from build123d import *

# Parameters (mm, degrees)
SKETCH1_W           = 52
SKETCH1_H           = 25
BOSS_EXTRUDE1_DEPTH = 2
SKETCH3_R           = 4
SKETCH3_R_2         = 1.5
CUT_EXTRUDE1_DEPTH  = 3
SKETCH4_R           = 4
SKETCH4_R_2         = 1.5
BOSS_EXTRUDE3_DEPTH = 2
SKETCH5_R           = 4
SKETCH5_R_2         = 1.496339982
SKETCH5_R_3         = 1.5
BOSS_EXTRUDE4_DEPTH = 2


with BuildPart() as part:
    # Sketch1 → Boss-Extrude1 (new body)
    with BuildSketch(Plane(origin=(0, 0, 0), x_dir=(1, 0, 0), z_dir=(0, 1, 0))):
        Rectangle(SKETCH1_W, SKETCH1_H)
    extrude(amount=BOSS_EXTRUDE1_DEPTH)

    # Sketch3 → Cut-Extrude1 (cut, through all)
    with BuildSketch(Plane(origin=(0, 2, 0), x_dir=(1, 0, 0), z_dir=(0, 1, 0))):
        Circle(SKETCH3_R)
        with Locations((18.6, 0)):
            Circle(SKETCH3_R_2)
        with Locations((7, 0)):
            Circle(SKETCH3_R_2)
        with Locations((0, 7)):
            Circle(SKETCH3_R_2)
        with Locations((-7, 0)):
            Circle(SKETCH3_R_2)
        with Locations((0, -7)):
            Circle(SKETCH3_R_2)
        with Locations((-18.6, 0)):
            Circle(SKETCH3_R_2)
    extrude(amount=-CUT_EXTRUDE1_DEPTH, mode=Mode.SUBTRACT)

    # Sketch4 → Boss-Extrude3 (add)
    with BuildSketch(Plane(origin=(26, 0, 0), x_dir=(0, 0, -1), z_dir=(1, 0, 0))):
        with BuildLine():
            Line((-12.5, 0), (12.5, 0))
            Line((12.5, 0), (12.5, 32))
            ThreePointArc((12.5, 32), (0, 44.5), (-12.5, 32))
            Line((-12.5, 32), (-12.5, 0))
        make_face()
        with Locations((0, 32)):
            Circle(SKETCH4_R, mode=Mode.SUBTRACT)
        with Locations((0, 39)):
            Circle(SKETCH4_R_2, mode=Mode.SUBTRACT)
        with Locations((7, 32)):
            Circle(SKETCH4_R_2, mode=Mode.SUBTRACT)
        with Locations((0, 25)):
            Circle(SKETCH4_R_2, mode=Mode.SUBTRACT)
        with Locations((-7, 32)):
            Circle(SKETCH4_R_2, mode=Mode.SUBTRACT)
        with Locations((0, 13.4)):
            Circle(SKETCH4_R_2, mode=Mode.SUBTRACT)
    extrude(amount=BOSS_EXTRUDE3_DEPTH)

    # Sketch5 → Boss-Extrude4 (add)
    with BuildSketch(Plane.ZY.offset(26)):
        with BuildLine():
            Line((-12.5, 0), (12.5, 0))
            Line((12.5, 0), (12.5, 32))
            ThreePointArc((12.5, 32), (0, 44.5), (-12.5, 32))
            Line((-12.5, 32), (-12.5, 0))
        make_face()
        with Locations((0, 32)):
            Circle(SKETCH5_R, mode=Mode.SUBTRACT)
        with Locations((0, 39)):
            Circle(SKETCH5_R_2, mode=Mode.SUBTRACT)
        with Locations((7, 32)):
            Circle(SKETCH5_R_3, mode=Mode.SUBTRACT)
        with Locations((0, 25)):
            Circle(SKETCH5_R_3, mode=Mode.SUBTRACT)
        with Locations((-7, 32)):
            Circle(SKETCH5_R_3, mode=Mode.SUBTRACT)
        with Locations((0, 13.4)):
            Circle(SKETCH5_R_3, mode=Mode.SUBTRACT)
    extrude(amount=BOSS_EXTRUDE4_DEPTH)


solid = part.part
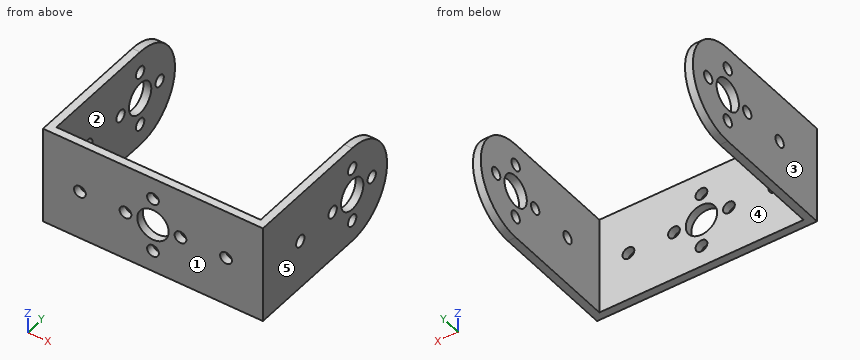
Could you check a few things on this model? Use its own coordinates, in mm. Face numbers are marked on the shaded views. A direction names the side the tool comes from. Give positions to 0.01 mm unless a question says otherwise; leave off trailing zeros. Order: outer loops, then holes, each group sorted by start corner. A loop starts at its lowest first (then second) coordinate and runs counter-clockwise, first axis right, second up. Notation, with made-up numbers: (47.5, 6.25) - (82.5, 6.25) arc R8 ccw to (82.5, 20.25) - close; hole circle Ø1 at (11, 58). An arc over 180 degrees is marked (long way). One line per question, with ' | ' between items. Start each with the question number.
Item 1: Thinking about a two-plate mould opening in X: for the marked faces 1, 2 and 3, which applies, pulls with the +X half, pulls with the -X half, needs draft (parallel to the pull), parting line crosses it, or undercut?
Item 2: For the marked faces 4 and 5, which set-ups out of +Z, -Z, +X, -X, +Y, -Y let a thin tool reach every point of the face, with its end or its side?
Item 3: I want a section at B-B on x = -18.6. Write out the boundary of the cut face in (y, z), then the cut area to 3 significant figures.
Item 4: I need wall thicknesses on probe 1 along Z at (x, y) = (0, 0.65); probe 2 along X at (y, z) = (16.5, -3); probe 3 along X at (y, z) = (1.55, -7). Which ranges of each line are inside material? Lowest first, please. Write a range as [from, to].
Item 5: I'm going to push flat-ended pins straight in: pin 1 Ø2.5 at (x, z) = (-7, 0) entering from -Y; pin 2 Ø3.5 at (x, z) = (7, 0) entering from +Y. Where does each tip first touch, or does it pass through?
Item 6: I want a section at D-D on z = 3. Write out the boundary of the cut face in (x, y).
Item 7: I want a section at C-C on y = 13.4. Write out the boundary of the cut face in (x, z).
Item 8: I want a section at A-A on y = 5. Write out the boundary of the cut face in (x, z), then the cut area to 3 significant figures.
Verdict:
1) face 1: needs draft | face 2: undercut | face 3: pulls with the -X half
2) face 4: +Z, -Z, +Y | face 5: +Z, -Z, +X, +Y, -Y
3) outline: (0, -12.5) - (2, -12.5) - (2, -1.5) - (0, -1.5) - close; (0, 1.5) - (2, 1.5) - (2, 12.5) - (0, 12.5) - close | area: 44.0 mm^2
4) probe 1: [-12.5, -8.5], [-5.5, -4], [4, 5.5], [8.5, 12.5] | probe 2: [-28, -26], [26, 28] | probe 3: [-28, -1.5], [1.5, 28]
5) pin 1: through | pin 2: y = 2
6) outline: (-28, 0) - (-2.65, 0) - (-2.65, 2) - (-26, 2) - (-26, 29.35) - (-28, 29.35) - close; (-28, 34.65) - (-26, 34.65) - (-26, 44.13) - (-28, 44.13) - close; (2.65, 0) - (28, 0) - (28, 29.35) - (26, 29.35) - (26, 2) - (2.65, 2) - close; (26, 34.65) - (28, 34.65) - (28, 44.13) - (26, 44.13) - close
7) outline: (-28, -12.5) - (-26, -12.5) - (-26, -1.5) - (-28, -1.5) - close; (-28, 1.5) - (-26, 1.5) - (-26, 12.5) - (-28, 12.5) - close; (26, -12.5) - (28, -12.5) - (28, -1.5) - (26, -1.5) - close; (26, 1.5) - (28, 1.5) - (28, 12.5) - (26, 12.5) - close
8) outline: (-28, -12.5) - (-26, -12.5) - (-26, 12.5) - (-28, 12.5) - close; (26, -12.5) - (28, -12.5) - (28, 12.5) - (26, 12.5) - close | area: 100 mm^2
